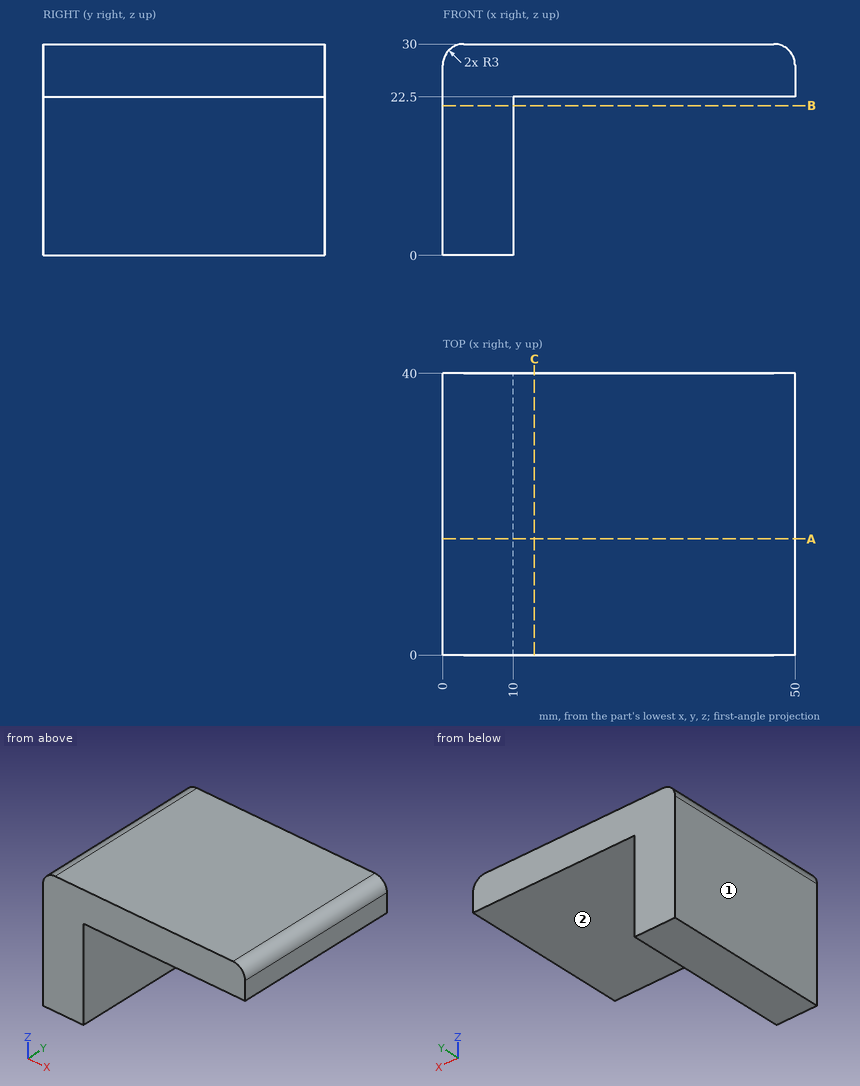
Study the drawing (mm; zero at the part's minimum x, y, z) and answer. A direction names the side the tool comes from. Round coordinates to 2 decimals unless told otherwise and drop trailing zeros. Write each loop counter-clockwise with the first axis right and the second up, starting at its lowest first coordinate (ties: lowest second). Pieces come first, ordered by that corner, then holes. Notation, with made-up numbers: (79, -34) - (93, -34) arc R15 cw to (93, -24) - close; hole circle Ø2 at (78.5, 87.5). An arc over 180 degrees is marked (long way). Use CSV: the item, a comma, the result in double quotes.
Q1. This flat-tipped pin is pushed along its axis until it touches: pin 1 Ø1.5 at (x, y) = (43.5, 14) entering from -Z. Where does it stop, or does it pass through?
Values:
pin 1,"stops at z = 22.5"
Q2. Find section A-A, the plane y = 16.5. Write down the section's boundary in (x, z), then the cut area to 3 significant figures.
Values:
outline,"(0, 0) - (10, 0) - (10, 22.5) - (50, 22.5) - (50, 27) arc R3 ccw to (47, 30) - (3, 30) arc R3 ccw to (0, 27) - close"
area,"596 mm²"
Q3. Straight lines are drawn through the part: line 1 along X through (y, z) = (25.5, 10); line 2 along Z through (x, y) = (42, 34.5). For each, find the intervals that lie inside material, in ascending order.
Values:
line 1,"x = 0 to 10"
line 2,"z = 22.5 to 30"
Q4. Find section B-B, the plane z = 21.25. Write down the section's boundary in (x, y).
Values:
outline,"(0, 0) - (10, 0) - (10, 40) - (0, 40) - close"
Q5. Find section C-C, the plane x = 13. Write down the section's boundary in (y, z), then the cut area to 3 significant figures.
Values:
outline,"(0, 22.5) - (40, 22.5) - (40, 30) - (0, 30) - close"
area,"300 mm²"
Q6. A tool of negligible diameter and unlimited length cuts with its end or side. For the marked faces 1 and 2, from which of +Z, -Z, +X, -X, +Y, -Y can it reach the whole face along a straight path? Write none if from no direction.
Values:
face 1,"+Z, -Z, -X, +Y, -Y"
face 2,"-Z, +X, +Y, -Y"
